```python
from build123d import *

# Parameters (mm, degrees)
BOSS_EXTRUDE1_DEPTH     = 5
CUT_EXTRUDE1_REACH      = 10.572
CUT_EXTRUDE1_END_RADIUS = 3.95
SKETCH2_R               = 1.55


with BuildPart() as part:
    # Sketch1 → Boss-Extrude1 (new, symmetric)
    with BuildSketch(Plane.XY):
        with BuildLine():
            Line((-3.533271058, -6), (3.533271058, -6))
            Line((3.533271058, -6), (3.533271058, 0))
            ThreePointArc((3.533271058, 0), (0, -2.184073719), (-3.533271058, 0))
            Line((-3.533271058, 0), (-3.533271058, -6))
        make_face()
    extrude(amount=BOSS_EXTRUDE1_DEPTH, both=True)

    # Cut-Extrude1: up to this cylinder (the profile starts outside it)
    cut_extrude1_end = Plane(origin=(0, 1.765926281, 0), z_dir=(0, 0, -1)) * Cylinder(CUT_EXTRUDE1_END_RADIUS, 30.044, mode=Mode.PRIVATE)
    # Sketch2 → Cut-Extrude1 (cut, up to the surface)
    with BuildSketch(Plane(origin=(0, -6, 0), x_dir=(-1, 0, 0), z_dir=(0, -1, 0)), mode=Mode.PRIVATE) as cut_extrude1_sk1:
        with Locations(Location((0, 0, 0), (0, 0, 90))):
            Circle(SKETCH2_R)
    cut_extrude1_tool1 = extrude(cut_extrude1_sk1.sketch, amount=-CUT_EXTRUDE1_REACH, mode=Mode.PRIVATE) - cut_extrude1_end
    add(cut_extrude1_tool1.solids().sort_by_distance((0, -6, 0))[0], mode=Mode.SUBTRACT)


solid = part.part
```
Read the model definition and answer for the solid it produces. Units are mm, in the model's axes. Give positions to 0.01 mm unless a question says otherwise; leave off trailing zeros. Loops run counter-clockwise (first coordinate to the right, second up) from the corner with the lowest first, then second, coordinate; pieces in that order, holes last.
Item 1: The part is cut by section B-B (x = 0). Write down the section's boundary in (y, z), and give its area (3 significant figures).
Item 2: The part is cut by section C-C (y = -2.5). Write down the section's boundary in (x, z), and give its area (3 significant figures).
Item 3: The mould has two halves that part along X. Classify faces 1 (the flat face through (0, -4, -5)), 2 (the cylindrical face through (0.07, -3.96, 1.55)), 3 (the flat face through (3.533, -3, 0)): released by +X, released by -X, zero draft, split by the parting line, or undercut.
Item 4: Find the intervals of material crossed by line 1 along Z through (x, y) = (0, -2.75); line 2 along X through (y, z) = (-4.4, 0); line 3 along X through (y, z) = (-5.25, 0.75), in increasing order.
Item 5: The part is cut by section A-A (z = 0). Write down the section's boundary in (x, y).
Item 6: The part is cut by section D-D (z = 3.5). Write down the section's boundary in (x, y).
Taken from the geometry:
1. outline: (-6, -5) - (-2.18, -5) - (-2.18, -1.55) - (-6, -1.55) - close; (-6, 1.55) - (-2.18, 1.55) - (-2.18, 5) - (-6, 5) - close
1. area: 26.3 mm2
2. outline: (-3.53, -5) - (3.53, -5) - (3.53, 5) - (-3.53, 5) - close; hole circle Ø3.1 at (0, 0)
2. area: 63.1 mm2
3. face 1: zero draft
3. face 2: undercut
3. face 3: released by +X
4. line 1: z = -5 to -1.55, 1.55 to 5
4. line 2: x = -3.53 to -1.55, 1.55 to 3.53
4. line 3: x = -3.53 to -1.36, 1.36 to 3.53
5. outline: (-3.53, -6) - (-1.55, -6) - (-1.55, -1.87) arc R3.95 cw to (-3.53, 0) - close; (1.55, -6) - (3.53, -6) - (3.53, 0) arc R3.95 cw to (1.55, -1.87) - close
6. outline: (-3.53, -6) - (3.53, -6) - (3.53, 0) arc R3.95 cw to (-3.53, 0) - close
